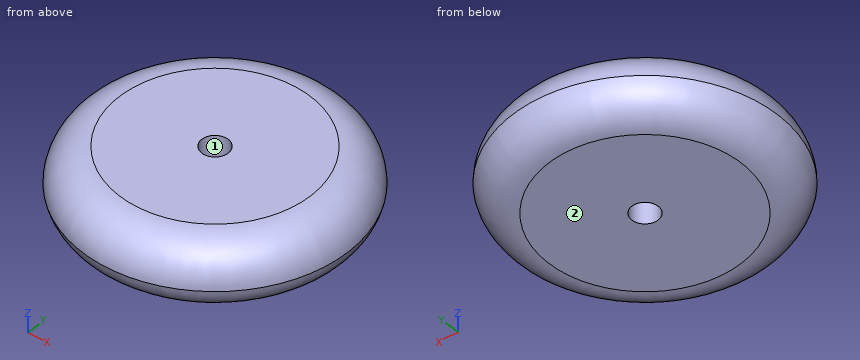
```python
from build123d import *

# Parameters (mm, degrees)
F2_R = 2.7869198521


# Not quite as in the source:
# - a fillet or chamfer that OpenCascade refuses, or shapes differently, is made with other operations: its cross-section is extruded or revolved along the edge and cut away or added


with BuildPart() as f1:
    # F0 (on Front) → F1 (revolve)
    with BuildSketch(Plane.XZ):
        Polygon((8.5, -2.5), (10, -2.5), (10, 2.5), (8.5, 2.5), (1, 2.5), (1, -2.5), align=None)
    revolve(axis=Axis((0, 0, 0), (0, 0, -1)))

    # F2
    f2_edges = [f1.edges().sort_by_distance(p)[0] for p in [
        (-10, 0, 2.5),
    ]]
    fillet(f2_edges, radius=F2_R)

    # F3: fillet of radius 2.787 on 1 edges, made by hand

    # F3_s1 → F3_t2 (revolve, cut)
    with BuildSketch(Plane.XZ):
        with BuildLine():
            ThreePointArc((10, -0.2869198521), (9.0288444344, -1.8771261086), (7.2727330524, -2.5))
            Line((7.2727330524, -2.5), (10, -2.5))
            Line((10, -2.5), (10, -0.2869198521))
        make_face()
    revolve(axis=Axis((0, 0, -2.5), (0, 0, -1)), mode=Mode.SUBTRACT)


solid = f1.part
```
Verification items for the finished model (mm, model axes). Face numbers are marked on the shaded views. Give positions to 0.01 mm unless a question says otherwise; leave off trailing zeros. Order: outer loops, then holes, each group sorted by start corner. A loop starts at its lowest first (then second) coordinate and runs counter-clockwise, first axis right, second up. Notation, with made-up numbers: (47, 16) -> (53, 16) arc R22 cw to (53, 42) -> close; hole circle Ø3 at (37, 84). An arc over 180 degrees is marked (long way). One line per item, written item: value.
(1) Sectioned sample at B-B on z = 2.2. Record the cut outline in (x, y), then the cut area to 3 significant figures.
Final values:
outline: circle Ø16.94 at (0, 0); hole circle Ø2 at (0, 0)
area: 222 mm^2
(2) Sectioned sample at A-A on x = 0. Record the cut outline in (y, z).
Final values:
outline: (-10, -0.29) arc R2.79 ccw to (-7.27, -2.5) -> (-1, -2.5) -> (-1, 2.5) -> (-7.21, 2.5) arc R2.79 ccw to start; (1, -2.5) -> (7.27, -2.5) arc R2.79 ccw to (10, -0.29) arc R2.79 ccw to (7.21, 2.5) -> (1, 2.5) -> close
(3) Draft check along X on the marked faces 1 and 2. Enter one of: pulls with the +X half, pulls with the -X half, needs draft (parallel to the pull), parting line crosses it, or undercut.
Final values:
face 1: undercut
face 2: needs draft
(4) Scan lines: line 1 along Y through (x, z) = (0, -0.3); line 2 along X through (y, z) = (0, 1.3); line 3 along X through (y, z) = (0, -0.6). Record each from-to range of solid material in increasing order. Write a range as [from, to].
Final values:
line 1: [-10, -1], [1, 10]
line 2: [-9.5, -1], [1, 9.5]
line 3: [-9.91, -1], [1, 9.91]
(5) Gauge pin test, flat ends, axial feed: pin 1 (2 mm diameter, centred on x = -4, z = 1.5, fed in from -Y); pin 2 (1.5 mm diameter, centred on y = -4.5, z = -0.5, fed in from +X). Record the tip position at first contact, or that the pin passes through.
Final values:
pin 1: y = -9.21
pin 2: x = 9.26
(6) Sectioned sample at C-C on z = -0.7. Record the cut outline in (x, y), then the cut area to 3 significant figures.
Final values:
outline: circle Ø19.76 at (0, 0); hole circle Ø2 at (0, 0)
area: 303 mm^2
